Part print with two shaded views. Sizes in mm from the minimum x, y, z corner. A direction names the side the tool comes from. Round coordinates to 2 decimals unless told otherwise and drop trailing zeros. Order: outer loops, then holes, each group sorted by start corner. A loop starts at its lowest first (then second) coordinate and runs counter-clockwise, first axis right, second up. Notation, with made-up numbers: (56.25, 47.25) - (63.25, 47.25) arc R32 cw to (63.25, 73.25) - close; hole circle Ø5 at (-10.5, -4.75). An arc over 180 degrees is marked (long way). Use one line per item in the form item = value.
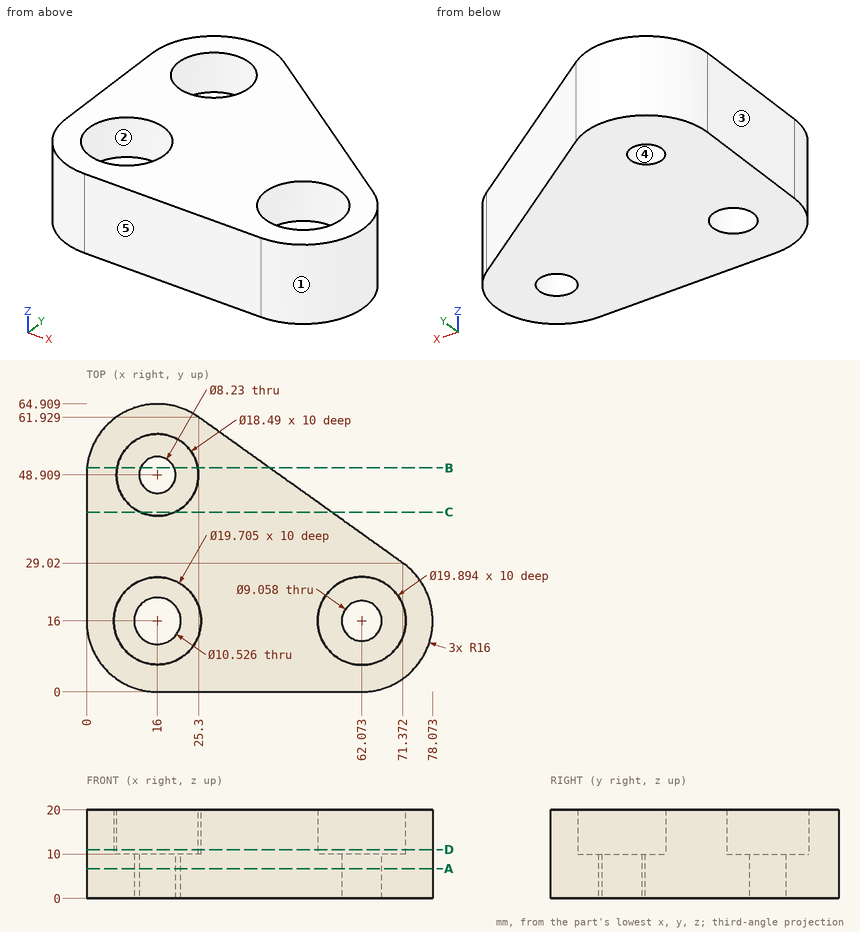
(1) Pin check, flat tips, straight feed: pin 1 (10 mm diameter, centred on y = 10.5, z = 11, fed in from +X) (1 decimal); pin 2 (5.5 mm diameter, centred on x = 13, y = 45.5, fed in from +Z); pin 3 (4 mm diameter, centred on x = 55, z = 3, fed in from +Y). Stop position of each tip, or through.
Report:
pin_1 = 78.1
pin_2 = 10
pin_3 = 42.14
(2) Probe probe 1 along X at (y, z) = (16, 16.75) (1 decimal); probe 2 along Y at (x, z) = (16, 15.25) (1 decimal); probe 3 along X at (y, z) = (17, 17.5) (1 decimal). List the from-to ranges inside material, lowest first. Write a range as [from, to].
Report:
probe_1 = [0, 6.1], [25.9, 52.1], [72, 78.1]
probe_2 = [0, 6.1], [25.9, 39.7], [58.2, 64.9]
probe_3 = [0, 6.2], [25.8, 52.2], [72, 78]
(3) Pull direction Y, two halves, no side cores. Call the marked faces 3, 4 and 5: released by +Y, released by -Y, zero draft, split by the parting line, or undercut.
Report:
face_3 = zero draft
face_4 = undercut
face_5 = released by -Y
(4) Slice it at C-C on y = 40.5. Give the cut face in (x, z).
Report:
outline = (0, 0) - (55.3, 0) - (55.3, 20) - (19.84, 20) - (19.84, 10) - (12.16, 10) - (12.16, 20) - (0, 20) - close
(5) Slice it at D-D on z = 11. Give the cut face in (x, y) (1 decimal).
Report:
outline = (0, 16) arc R16 ccw to (16, 0) - (62.1, 0) arc R16 ccw to (71.4, 29) - (25.3, 61.9) arc R16 ccw to (0, 48.9) - close; hole circle Ø19.7 at (16, 16); hole circle Ø18.5 at (16, 48.9); hole circle Ø19.9 at (62.1, 16)
(6) Tool access for the marked faces 1 and 2: list every direction of +Z, -Z, +X, -X, +Y, -Y with a clear straight run to the whole face (end or side of a thin tool).
Report:
face_1 = +Z, -Z, +X
face_2 = +Z
(7) Slice it at A-A on z = 6.75. Give the cut face in (x, y) (1 decimal).
Report:
outline = (0, 16) arc R16 ccw to (16, 0) - (62.1, 0) arc R16 ccw to (71.4, 29) - (25.3, 61.9) arc R16 ccw to (0, 48.9) - close; hole circle Ø10.5 at (16, 16); hole circle Ø8.2 at (16, 48.9); hole circle Ø9.1 at (62.1, 16)
(8) Slice it at B-B on y = 50.5. Give the cut face in (x, z) (1 decimal).
Report:
outline = (0.1, 0) - (12.2, 0) - (12.2, 10) - (6.9, 10) - (6.9, 20) - (0.1, 20) - close; (19.8, 0) - (41.3, 0) - (41.3, 20) - (25.1, 20) - (25.1, 10) - (19.8, 10) - close
